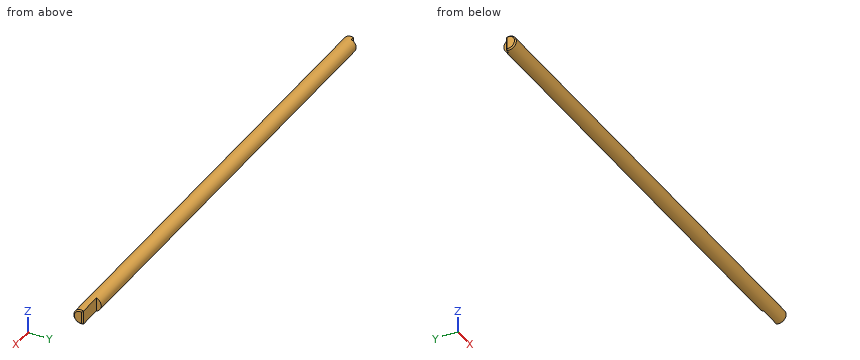
from build123d import *

# Parameters (mm, degrees)
SKETCH1_W               = 200
SKETCH1_H               = 3
CUT_EXTRUDE1_DEPTH      = 201.044994939
CUT_EXTRUDE1_DEPTH_BACK = 201.044994939
SKETCH2_W               = 2
SKETCH2_H               = 2
SKETCH2_W_2             = 10
CHAMFER1_SIZE           = 0.5


with BuildPart() as part:
    # Sketch1 → Revolve1 (revolve)
    with BuildSketch(Plane.XY, mode=Mode.PRIVATE) as revolve1_sk:
        with Locations((100, 1.5)):
            Rectangle(SKETCH1_W, SKETCH1_H)
    revolve(revolve1_sk.sketch.rotate(Axis((0, 0, 0), (1, 0, 0)), 90), axis=Axis((0, 0, 0), (1, 0, 0)))

    # Sketch2 → Cut-Extrude1 (cut, two sides: drawn at the far end of the back side and taken through both)
    with BuildSketch(Plane.XY.offset(-CUT_EXTRUDE1_DEPTH_BACK)):
        with Locations((1, 2)):
            Rectangle(SKETCH2_W, SKETCH2_H)
        with Locations((195, 2)):
            Rectangle(SKETCH2_W_2, SKETCH2_H)
    extrude(amount=CUT_EXTRUDE1_DEPTH + CUT_EXTRUDE1_DEPTH_BACK, mode=Mode.SUBTRACT)

    # Chamfer1
    chamfer1_edges = [part.edges().sort_by_distance(p)[0] for p in [
        (0, 1, 0),
        (200, -2.956795679, -0.507305936),
        (200, 1, 0),
        (0, -2.956795679, -0.507305936),
    ]]
    chamfer(chamfer1_edges, length=CHAMFER1_SIZE)


solid = part.part
Part model, mm, in its own coordinate system. Coordinates: 2 decimals unless noted, no trailing zeros. Loops run counter-clockwise (first coordinate to the right, second up) from the corner with the lowest first, then second, coordinate; pieces in that order, holes last. Notation, with made-up numbers: M 15,73.5 L 52,73.5 A9 ccw 52,83.5 Z; hole C 30.25,73 d10. An arc over 180 degrees is marked long. Use a Markdown table: item, result. Add a question column.
Q1. Cut at B-B (x = 70.5). Write the cut outline in (y, z), and give its area (3 significant figures).
Q2. Cut at A-A (z = 0). Write the cut outline in (x, y).
Q3. Probe L1, parallel to Y at x = 46, z = 0.25; L2, parallel to Z at x = 145, y = -1; L3, parallel to X at y = 1.7, z = 0.15. List the from-to ranges inside material, lowest first.
Q4. Pin check, flat tips, straight feed: P1, Ø3, axis at x = 194, z = -1, coming from the +Y side; P2, Ø0.6, axis at y = 1.5, z = 0, coming from the -X side; P3, Ø1, axis at x = 33, y = 1.5, coming from the -Z side. Stop position of each tip, or through.
Worked out:
| question | item | result |
|---|---|---|
| 1 | outline | C 0,0 d6 |
| 1 | area | 28.3 mm2 |
| 2 | outline | M 0,-2.5 L 0.5,-3 L 199.5,-3 L 200,-2.5 L 200,0.5 L 199.5,1 L 190,1 L 190,3 L 2,3 L 2,1 L 0.5,1 L 0,0.5 Z |
| 3 | L1 | y = -2.99 to 2.99 |
| 3 | L2 | z = -2.83 to 2.83 |
| 3 | L3 | x = 2 to 190 |
| 4 | P1 | stops at y = 1 |
| 4 | P2 | stops at x = 2 |
| 4 | P3 | stops at z = -2.83 |
